from build123d import *

# Parameters (mm, degrees)
F0_W     = 38
F0_H     = 10
F0_R     = 1.9
F1_DEPTH = 10
F2_W     = 18
F2_H     = 3
F3_DEPTH = 10.001
F4_R     = 2.7
F5_DEPTH = 4
F6_R     = 2
F7_R     = 4
F8_DEPTH = 3


with BuildPart() as f1:
    # F0 (on Top) → F1 (new body)
    with BuildSketch(Plane.XY):
        Rectangle(F0_W, F0_H)
        with Locations((-14.15, 0)):
            Circle(F0_R, mode=Mode.SUBTRACT)
        with Locations((14.15, 0)):
            Circle(F0_R, mode=Mode.SUBTRACT)
    extrude(amount=F1_DEPTH)

    # F2 (on face) → F3 (cut, through all)
    with BuildSketch(Plane.XZ.offset(5)):
        with Locations((0, 1.5)):
            Rectangle(F2_W, F2_H)
    extrude(amount=-F3_DEPTH, mode=Mode.SUBTRACT)

    # F4 (on face) → F5 (cut)
    with BuildSketch(Plane(origin=(0, 0, 0), x_dir=(1, 0, 0), z_dir=(0, 0, -1))):
        with Locations((-14.15, 0)):
            Circle(F4_R)
        with Locations((14.15, 0)):
            Circle(F4_R)
    extrude(amount=-F5_DEPTH, mode=Mode.SUBTRACT)

    # F6
    f6_edges = [f1.edges().sort_by_distance(p)[0] for p in [
        (-9, 0, 3),
        (9, 0, 3),
    ]]
    fillet(f6_edges, radius=F6_R)

    # F7 (on face) → F8 (cut)
    with BuildSketch(Plane.XY.offset(10)):
        with Locations((-14.15, 0)):
            Circle(F7_R)
        with Locations((14.15, 0)):
            Circle(F7_R)
    extrude(amount=-F8_DEPTH, mode=Mode.SUBTRACT)


solid = f1.part
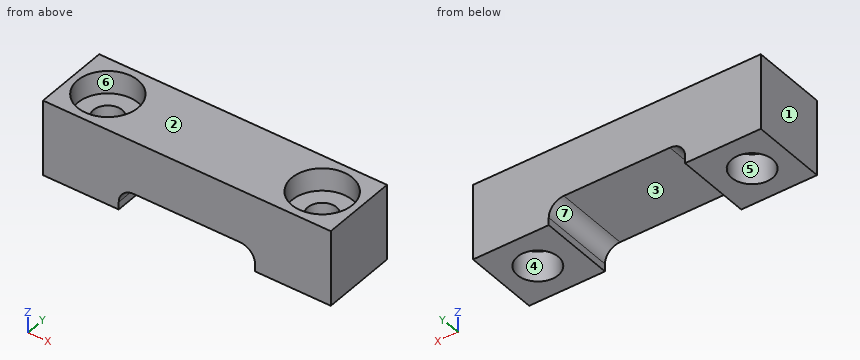
Geometry: final body of the model. Coordinates: model frame, mm. Face numbers are marked on the shaded views. A direction names the side the tool comes from. Round coordinates to 2 decimals unless told otherwise and drop trailing zeros. Loops run counter-clockwise (first coordinate to the right, second up) from the corner with the lowest first, then second, coordinate; pieces in that order, holes last.
Q1. Section A-A on y = 0. State how many separate pieces and enclosed holes the cut face has, plus the area to 3 significant figures.
Q2. Section D-D on x = -5. Return loops of the section in (y, z).
Q3. Access query for the marked faces 5, 6 and 7. Directions: +Z, -Z, +X, -X, +Y, -Y. A direction counts if a zero-diameter tool reaches every point of the face in a straight line with its end or side. Return the directions, or none.
Q4. Section B-B on x = 14.15. Return loops of the section in (y, z).
Q5. Pull-direction query (X, two-part tool) for the marked faces 1, 2, 3 and 4; classes: released by +X, released by -X, zero draft, split by the parting line, or undercut.
Q6. Pin query (flat end, axial travel): P1, Ø4.5, axis at x = -14.15, y = 0, coming from the -Z side; P2, Ø2.5, axis at x = -13, y = 2, coming from the +Z side; P3, Ø5, axis at x = 1, y = 1, coming from the -Z side; P4, Ø1.6, axis at x = -14, y = 1, coming from the -Z side. Return the tip coordinate at first contact, or that it passes through.
Q7. Material intervals for L1, parallel to X at y = 0, z = 5.4; L2, parallel to Y at x = 14.15, z = 1; L3, parallel to Y at x = 14.15, z = 4.8, sorted ascending.
Q8. Section C-C on z = 9. Return loops of the section in (x, y), plus the area to 3 significant figures.
Evaluation:
1. separate pieces: 3
1. enclosed holes: 0
1. area: 214 mm2
2. outline: (-5, 3) - (5, 3) - (5, 10) - (-5, 10) - close
3. face 5: -Z
3. face 6: +Z
3. face 7: -Z, +Y, -Y
4. outline: (-5, 0) - (-2.7, 0) - (-2.7, 4) - (-1.9, 4) - (-1.9, 7) - (-4, 7) - (-4, 10) - (-5, 10) - close; (1.9, 4) - (2.7, 4) - (2.7, 0) - (5, 0) - (5, 10) - (4, 10) - (4, 7) - (1.9, 7) - close
5. face 1: released by -X
5. face 2: zero draft
5. face 3: undercut
5. face 4: undercut
6. P1: stops at z = 4
6. P2: stops at z = 7
6. P3: stops at z = 3
6. P4: passes through
7. L1: x = -19 to -16.05, -12.25 to 12.25, 16.05 to 19
7. L2: y = -5 to -2.7, 2.7 to 5
7. L3: y = -5 to -1.9, 1.9 to 5
8. outline: (-19, -5) - (19, -5) - (19, 5) - (-19, 5) - close; hole circle Ø8 at (-14.15, 0); hole circle Ø8 at (14.15, 0)
8. area: 279 mm2
